Read the model definition and answer for the solid it produces. Units are mm, in the model's axes. Give positions to 0.01 mm unless a question says otherwise; leave off trailing zeros. Loops run counter-clockwise (first coordinate to the right, second up) from the corner with the lowest first, then second, coordinate; pieces in that order, holes last. Notation, with made-up numbers: (-23, -37) -> (6, -37) arc R22 cw to (6, -31) -> close; hole circle Ø1 at (2.25, 87.5). An arc over 180 degrees is marked (long way). Return JSON: item names as keys, results as strings. Group by question number.
Autodesk Inventor part; units mm, degrees
ref_plane "YZ Plane" through (0, 0, 0) normal (1, 0, 0) x (0, 1, 0)
ref_plane "XZ Plane" through (0, 0, 0) normal (0, 1, 0) x (-1, 0, 0)
ref_plane "XY Plane" through (0, 0, 0) normal (0, 0, 1) x (1, 0, 0)
sketch "Boceto1" plane through (0, 0, 0) normal (0, 0, 1) x (1, 0, 0)
  line L0 (40, 70) -> (40, 5)
  line L1 (2.5, 60) -> (7.5, 60)
  line L2 (7.5, 60) -> (7.5, 5)
  line L3 (7.5, 5) -> (2.5, 5)
  line L4 (2.5, 5) -> (2.5, 60)
  line L5 (12.5, 60) -> (17.5, 60)
  line L6 (17.5, 60) -> (17.5, 5)
  line L7 (17.5, 5) -> (12.5, 5)
  line L8 (12.5, 5) -> (12.5, 60)
  line L9 (22.5, 60) -> (27.5, 60)
  line L10 (27.5, 60) -> (27.5, 5)
  line L11 (27.5, 5) -> (22.5, 5)
  line L12 (22.5, 5) -> (22.5, 60)
  line L13 (32.5, 60) -> (37.5, 60)
  line L14 (37.5, 60) -> (37.5, 5)
  line L15 (37.5, 5) -> (32.5, 5)
  line L16 (32.5, 5) -> (32.5, 60)
  line L17 (138.5, 90) -> (138.5, 0)
  line L18 (138.5, 0) -> (98.5, 0)
  line L19 (98.5, 0) -> (98.5, 70)
  line L20 (101, 60) -> (106, 60)
  line L21 (106, 60) -> (106, 5)
  line L22 (106, 5) -> (101, 5)
  line L23 (101, 5) -> (101, 60)
  line L24 (111, 60) -> (116, 60)
  line L25 (116, 60) -> (116, 5)
  line L26 (116, 5) -> (111, 5)
  line L27 (111, 5) -> (111, 60)
  line L28 (121, 60) -> (126, 60)
  line L29 (126, 60) -> (126, 5)
  line L30 (126, 5) -> (121, 5)
  line L31 (121, 5) -> (121, 60)
  line L32 (136, 60) -> (136, 5)
  line L33 (131, 5) -> (131, 60)
  line L34 (131, 60) -> (136, 60)
  line L35 (136, 5) -> (131, 5)
  line L36 (0, 90) -> (138.5, 90)
  line L37 (40, 70) -> (98.5, 70)
  line L38 (17.5, 78.25) -> (22.5, 78.25)
  line L39 (22.5, 78.25) -> (22.5, 75.25)
  line L40 (22.5, 75.25) -> (17.5, 75.25)
  line L41 (17.5, 75.25) -> (17.5, 78.25)
  line L42 (20, 78.25) -> (20, 75.25) construction
  line L43 (17.5, 76.75) -> (22.5, 76.75) construction
  line L44 (57.5, 78.25) -> (62.5, 78.25)
  line L45 (62.5, 78.25) -> (62.5, 75.25)
  line L46 (62.5, 75.25) -> (57.5, 75.25)
  line L47 (57.5, 75.25) -> (57.5, 78.25)
  line L48 (60, 78.25) -> (60, 75.25) construction
  line L49 (57.5, 76.75) -> (62.5, 76.75) construction
  line L50 (45, 0) -> (45, 5)
  line L51 (45, 5) -> (40, 5)
  line L52 (45, 0) -> (0, 0)
  line L53 (0, 78.25) -> (-12.5, 78.25)
  line L54 (-12.5, 78.25) -> (-12.5, 73.25)
  line L55 (-12.5, 73.25) -> (0, 73.25)
  line L56 (0, 0) -> (0, 73.25)
  line L57 (0, 78.25) -> (0, 90)
  point P0 (0, 0)
  dimension "d46" = 5
  dimension "d85" = 5
  dimension "d86" = 5
  dimension "d87" = 5
  dimension "d89" = 40
  dimension "d90" = 5
  dimension "d94" = 5
  dimension "d95" = 5
  dimension "d96" = 5
  dimension "d112" = 2.5
  dimension "d120" = 5
  dimension "d121" = 3
  dimension "d134" = 5
  dimension "d135" = 3
  dimension "d136" = 35
  dimension "d141" = 5
  dimension "d145" = 55
  dimension "d155" = 70
  dimension "d156" = 90
  dimension "d157" = 76.75
  dimension "d158" = 5
  dimension "d161" = 5
  dimension "d162" = 40
  dimension "d163" = 2.5
  dimension "d164" = 138.5
  dimension "d165" = 20
  dimension "d166" = 12.5
extrude "Extrusión7" add sketch "Boceto1" along normal blind 3
properties part number "Celda puertas"
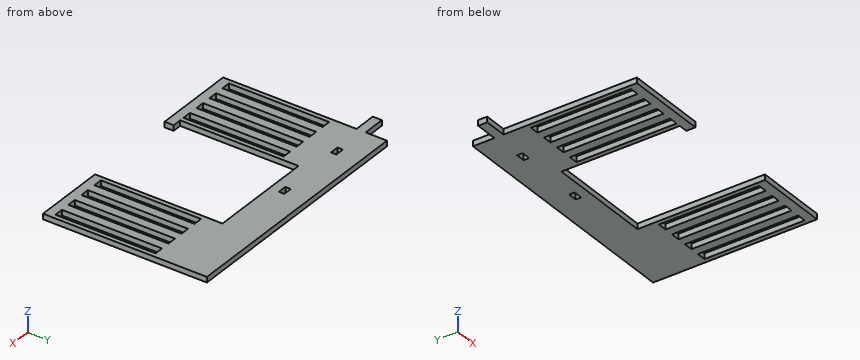
1. Section A-A on x = 4.5 is taken. Determine the outline of the cut face in (y, z), then the cut area to 3 significant figures.
2. Section C-C on y = 42 is taken. State how many separate pieces and enclosed holes the cut face has, then the cut area to 3 significant figures.
3. Flat-ended cylindrical pins translate along their axes: pin 1 Ø1.5 at (y, z) = (27.5, 2) entering from -X; pin 2 Ø1.5 at (x, z) = (-7, 1.5) entering from +Y. Find the tip coordinate at first contact, or state that the pin passes through.
4. Straight lines are drawn through the part: line 1 (Y direction, x = 37, z = 2.95); line 2 (Y direction, x = 20, z = 1.15); line 3 (Y direction, x = 80.5, z = 0.7). For each, find the intervals that lie inside material, in ascending order. Write a range as from..to.
5. Section B-B on y = 67.5 is taken. Determine the outline of the cut face in (x, z), then the cut area to 3 significant figures.
Completed:
{
 "1": {"outline": "(0, 0) -> (5, 0) -> (5, 3) -> (0, 3) -> close; (60, 0) -> (90, 0) -> (90, 3) -> (60, 3) -> close", "area": "105 mm²"},
 "2": {"separate pieces": "10", "enclosed holes": "0", "area": "120 mm²"},
 "3": {"pin 1": "stops at x = 0", "pin 2": "stops at y = 78.25"},
 "4": {"line 1": "y = 0..5, 60..90", "line 2": "y = 0..75.25, 78.25..90", "line 3": "y = 70..90"},
 "5": {"outline": "(0, 0) -> (40, 0) -> (40, 3) -> (0, 3) -> close; (98.5, 0) -> (138.5, 0) -> (138.5, 3) -> (98.5, 3) -> close", "area": "240 mm²"}
}
